Geometry: see drawing. Coordinates: mm, zero at the bounding-box minimum. A direction names the side the tool comes from. Give positions to 0.01 mm unless a question says otherwise; leave off trailing zeros. Order: outer loops, then holes, each group sorted by start corner. A loop starts at its lowest first (then second) coordinate and runs counter-clockwise, first axis right, second up. Notation, with made-up numbers: M 1.25,39.5 L 22.25,39.5 A31 ccw 22.25,78.5 Z; hole C 72.25,81.5 d9. An arc over 180 degrees is marked long. Use a Markdown table: item, result.
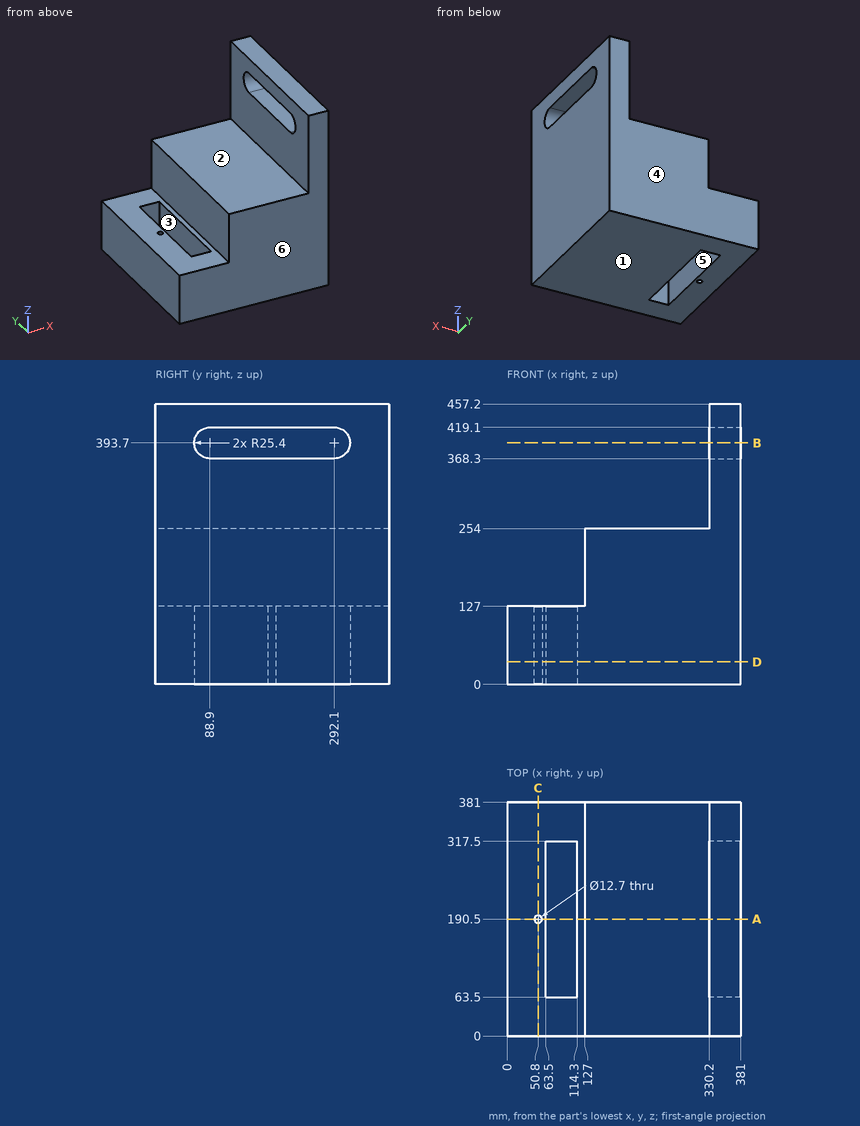
1) Material intervals for line 1 (X direction, y = 190, z = 43); line 2 (X direction, y = 198.5, z = 34.5); line 3 (Y direction, x = 50.8, z = 26), sorted ascending. Write a range as from..to.
Response values:
| item | result |
|---|---|
| line 1 | x = 0..44.47, 57.13..63.5, 114.3..381 |
| line 2 | x = 0..63.5, 114.3..381 |
| line 3 | y = 0..184.15, 196.85..381 |
2) Cut plane C-C on x = 50.8. Return loops of the section in (y, z), and give its area (3 significant figures).
Response values:
| item | result |
|---|---|
| outline | M 0,0 L 184.15,0 L 184.15,127 L 0,127 Z; M 196.85,0 L 381,0 L 381,127 L 196.85,127 Z |
| area | 46,800 mm² |
3) Mould query, pull axis Y, two halves, no side actions, for the marked faces 4, 5 and 6. Classes: released by +Y, released by -Y, zero draft, split by the parting line, or undercut.
Response values:
| item | result |
|---|---|
| face 4 | released by +Y |
| face 5 | undercut |
| face 6 | released by -Y |
4) Cut plane A-A on y = 190.5. Return loops of the section in (x, z), and give its area (3 significant figures).
Response values:
| item | result |
|---|---|
| outline | M 0,0 L 44.45,0 L 44.45,127 L 0,127 Z; M 57.15,0 L 63.5,0 L 63.5,127 L 57.15,127 Z; M 114.3,0 L 381,0 L 381,368.3 L 330.2,368.3 L 330.2,254 L 127,254 L 127,127 L 114.3,127 Z; M 330.2,419.1 L 381,419.1 L 381,457.2 L 330.2,457.2 Z |
| area | 80,300 mm² |
5) Cut plane D-D on z = 36.5. Return loops of the section in (x, y), and give its area (3 significant figures).
Response values:
| item | result |
|---|---|
| outline | M 0,0 L 381,0 L 381,381 L 0,381 Z; hole C 50.8,190.5 d12.7; hole M 63.5,63.5 L 114.3,63.5 L 114.3,317.5 L 63.5,317.5 Z |
| area | 132,000 mm² |
6) Cut plane B-B on z = 393.7. Return loops of the section in (x, y), and give its area (3 significant figures).
Response values:
| item | result |
|---|---|
| outline | M 330.2,0 L 381,0 L 381,63.5 L 330.2,63.5 Z; M 330.2,317.5 L 381,317.5 L 381,381 L 330.2,381 Z |
| area | 6,450 mm² |
7) Reachability of the marked faces 1, 2 and 3 from +Z, -Z, +X, -X, +Y, -Y: full face, straight path, thin tool, end or side. Return the list, or none.
Response values:
| item | result |
|---|---|
| face 1 | -Z, +X, -X, +Y, -Y |
| face 2 | +Z, -X, +Y, -Y |
| face 3 | +Z, -Z |
8) First-contact query: pin 1 Ø1 at (x, y) = (232, 40) entering from +Z; pin 2 Ø1 at (y, z) = (297.5, 324.5) entering from -X. Flat tips, straight axial feed; report the tip coordinate or a pass-through.
Response values:
| item | result |
|---|---|
| pin 1 | stops at z = 254 |
| pin 2 | stops at x = 330.2 |
